Verification items for the finished model (mm, model axes). A direction names the side the tool comes from. Round coordinates to 2 decimals unless told otherwise and drop trailing zeros. Loops run counter-clockwise (first coordinate to the right, second up) from the corner with the lowest first, then second, coordinate; pieces in that order, holes last. Notation, with made-up numbers: M -11.5,30.5 L -0.5,30.5 A11 ccw -0.5,49.5 Z; hole C -12.5,-27.5 d7. An arc over 180 degrees is marked long. Write item = value, one per line. Start each with the question number.
from build123d import *

# Parameters (mm, degrees)
BASE_FLANGE1_DEPTH = 88.9
CUT_EXTRUDE1_REACH = 101.653
SKETCH6_R          = 3.667750264
SKETCH6_W          = 11.0998
SKETCH6_H          = 50.8
FILLET2_R          = 3


# Sheet-metal steps are written as plain solids
with BuildPart() as part:
    # Sketch1 → Base-Flange1 (new body)
    with BuildSketch(Plane(origin=(0, 0, 0), x_dir=(1, 0, 0), z_dir=(0, 1, 0))):
        with BuildLine():
            Line((0, 0), (24.111, 0))
            ThreePointArc((24.111, 0), (24.739617928, 0.260382072), (25, 0.889))
            Line((25, 0.889), (25, 19.676430462))
            ThreePointArc((25, 19.676430462), (24.94638674, 19.980486369), (24.79201351, 20.247868647))
            Line((24.79201351, 20.247868647), (12.144247806, 35.320888862))
            Line((12.144247806, 35.320888862), (13.36034336, 36.341314193))
            Line((13.36034336, 36.341314193), (26.008109063, 21.268293977))
            ThreePointArc((26.008109063, 21.268293977), (26.438148775, 20.523443347), (26.5875, 19.676430462))
            Line((26.5875, 19.676430462), (26.5875, 0.889))
            ThreePointArc((26.5875, 0.889), (25.862149944, -0.862149944), (24.111, -1.5875))
            Line((24.111, -1.5875), (0, -1.5875))
            Line((0, -1.5875), (0, 0))
        make_face()
    extrude(amount=BASE_FLANGE1_DEPTH)

    # Sketch6 → Cut-Extrude1 (cut, up to next)
    with BuildSketch(Plane(origin=(26.5875, 0, 0), x_dir=(0, 0, -1), z_dir=(1, 0, 0)), mode=Mode.PRIVATE) as cut_extrude1_sk1:
        with Locations((7.889, 79.35)):
            Circle(SKETCH6_R)
    cut_extrude1_tool1 = extrude(cut_extrude1_sk1.sketch, amount=-CUT_EXTRUDE1_REACH, mode=Mode.PRIVATE) & part.part
    # Sketch6 → Cut-Extrude1 (cut, up to next)
    with BuildSketch(Plane(origin=(26.5875, 0, 0), x_dir=(0, 0, -1), z_dir=(1, 0, 0)), mode=Mode.PRIVATE) as cut_extrude1_sk2:
        with Locations((7.889, 9.5)):
            Circle(SKETCH6_R)
    cut_extrude1_tool2 = extrude(cut_extrude1_sk2.sketch, amount=-CUT_EXTRUDE1_REACH, mode=Mode.PRIVATE) & part.part
    # Sketch6 → Cut-Extrude1 (cut, up to next)
    with BuildSketch(Plane(origin=(26.5875, 0, 0), x_dir=(0, 0, -1), z_dir=(1, 0, 0)), mode=Mode.PRIVATE) as cut_extrude1_sk3:
        with Locations((7.897214616, 43.4059352)):
            Rectangle(SKETCH6_W, SKETCH6_H)
    cut_extrude1_tool3 = extrude(cut_extrude1_sk3.sketch, amount=-CUT_EXTRUDE1_REACH, mode=Mode.PRIVATE) & part.part
    add(cut_extrude1_tool1.solids().sort_by_distance((26.5875, 79.35, -7.889))[0], mode=Mode.SUBTRACT)
    add(cut_extrude1_tool2.solids().sort_by_distance((26.5875, 9.5, -7.889))[0], mode=Mode.SUBTRACT)
    add(cut_extrude1_tool3.solids().sort_by_distance((26.5875, 43.405935, -7.897215))[0], mode=Mode.SUBTRACT)

    # Fillet2
    fillet2_edges = [part.edges().sort_by_distance(p)[0] for p in [
        (25.79375, 68.8059352, -13.447114616),
        (25.79375, 18.0059352, -13.447114616),
        (25.79375, 18.0059352, -2.347314616),
        (25.79375, 68.8059352, -2.347314616),
    ]]
    fillet(fillet2_edges, radius=FILLET2_R)


solid = part.part
1. Section check A-A, the plane y = 33.5. Enter the section's corners in (x, z), and give its area (3 significant figures).
2. Mould release check, pull along Z, two halves, no side actions. Record for faces 4 (the flat face through (26, 43, -2.347)), 5 (the flat face through (19.596, 43.828, -28.91)), 6 (the flat face through (12, 44, 1.588)): pulls with the +Z half, pulls with the -Z half, needs draft (parallel to the pull), parting line crosses it, or undercut.
3. Section check D-D, the plane x = 5.25. Enter the section's corners in (y, z).
4. Section check C-C, the plane y = 9.5. Enter the section's corners in (x, z), and give its area (3 significant figures).
5. Gauge pin test, flat ends, axial feed: P1, Ø6, axis at y = 79, z = -30, coming from the -X side; P2, Ø7, axis at x = 12, y = 47.5, coming from the -Z side; P3, Ø9.5, axis at y = 66, z = -9, coming from the -X side; P4, Ø12, axis at x = 9, z = -8, coming from the -Y side. Record the tip position at first contact, or that the pin passes through.
6. Tool access check on faces 1 (the flat face through (26, 68.806, -8)), 2 (the flat face through (18.557, 43.828, -27.679)), 3 (the flat face through (25.2, 0, -11.8)). Record the directions out of +Z, -Z, +X, -X, +Y, -Y that give a thin tool (end or side, any length) a straight path to the whole face; none if there is none.
7. Section check B-B, the plane x = 19. Enter the section's corners in (y, z).
8. Thickness scan on line 1 (Z direction, x = 9.25, y = 25); line 2 (Z direction, x = 12.75, y = 43.5); line 3 (X direction, y = 61, z = -17). Record the ranges inside material, lowest first.
Computed values:
q1.outline = M 0,0 L 24.11,0 A0.89 cw 25,-0.89 L 25,-2.35 L 26.59,-2.35 L 26.59,-0.89 A2.48 ccw 24.11,1.59 L 0,1.59 Z; M 12.14,-35.32 L 13.36,-36.34 L 26.01,-21.27 A2.48 ccw 26.59,-19.68 L 26.59,-13.45 L 25,-13.45 L 25,-19.68 A0.89 cw 24.79,-20.25 Z
q1.area = 87.8 mm2
q2.face_4 = undercut
q2.face_5 = pulls with the -Z half
q2.face_6 = pulls with the +Z half
q3.outline = M 0,0 L 88.9,0 L 88.9,1.59 L 0,1.59 Z
q4.outline = M 0,0 L 24.11,0 A0.89 cw 25,-0.89 L 25,-4.22 L 26.59,-4.22 L 26.59,-0.89 A2.48 ccw 24.11,1.59 L 0,1.59 Z; M 12.14,-35.32 L 13.36,-36.34 L 26.01,-21.27 A2.48 ccw 26.59,-19.68 L 26.59,-11.56 L 25,-11.56 L 25,-19.68 A0.89 cw 24.79,-20.25 Z
q4.area = 93.8 mm2
q5.P1 = 14.09
q5.P2 = -36.34
q5.P3 = 25
q5.P4 = through
q6.face_1 = +X, -X
q6.face_2 = -X, +Y, -Y
q6.face_3 = +Z, -Z, +X, -X, -Y
q7.outline = M 0,-29.62 L 88.9,-29.62 L 88.9,-27.15 L 0,-27.15 Z; M 0,0 L 88.9,0 L 88.9,1.59 L 0,1.59 Z
q8.line_1 = 0 to 1.59
q8.line_2 = -35.83 to -34.6, 0 to 1.59
q8.line_3 = 25 to 26.59
